from build123d import *

# Parameters (mm, degrees)
F0_W      = 127
F0_H      = 127
F1_DEPTH  = 127
F2_DEPTH  = 25.4
F3_DEPTH  = 76.2
F5_DEPTH  = 228.6
F6_W      = 55.9784695506
F6_H      = 69.2825764418
F7_DEPTH  = 5.08
F8_W      = 69.8941033334
F8_H      = 56.1961345005
F9_DEPTH  = 7.62
F11_W     = 69.8941033334
F11_H     = 56.1961345005
F10_W     = 69.8941033334
F10_H     = 56.1961345005
F12_DEPTH = 7.62
F13_T     = -5.08


# Not quite as in the source:
# - a shell that OpenCascade refuses in one call is made with other operations: the cavity is built on its own and cut out


with BuildPart() as f1:
    # F0 (on Top) → F1 (new body)
    with BuildSketch(Plane.XY):
        with Locations((63.5, -63.5)):
            Rectangle(F0_W, F0_H)
    extrude(amount=F1_DEPTH)

    # F2 (add): a face of the model
    f2_faces = [f1.faces().sort_by_distance(p)[0] for p in [
        (63.5, -127, 63.5),
    ]]
    extrude(f2_faces, amount=F2_DEPTH)

    # F3 (add): a face of the model
    f3_faces = [f1.faces().sort_by_distance(p)[0] for p in [
        (63.5, -152.4, 63.5),
    ]]
    extrude(f3_faces, amount=F3_DEPTH)

    # F4 (on face) → F5 (join)
    with BuildSketch(Plane.XZ.offset(228.6)):
        Polygon((63.5, 210.3958427906), (63.5, 127), (127, 127), align=None)
        Polygon((63.5, 210.3958427906), (0, 127), (63.5, 127), align=None)
    extrude(amount=-F5_DEPTH)

    # F6 (on face) → F7 (cut)
    with BuildSketch(Plane.XZ.offset(228.6)):
        with Locations((68.3894939721, 34.6412882209)):
            Rectangle(F6_W, F6_H)
    extrude(amount=-F7_DEPTH, mode=Mode.SUBTRACT)

    # F8 (on face) → F9 (cut)
    with BuildSketch(Plane(origin=(0, 0, 0), x_dir=(0, -1, 0), z_dir=(-1, 0, 0))):
        with Locations((55.1468739286, 62.0407964849)):
            Rectangle(F8_W, F8_H)
        with Locations((160.0488739286, 62.0407964849)):
            Rectangle(F8_W, F8_H)
    extrude(amount=-F9_DEPTH, mode=Mode.SUBTRACT)

    # F11 (on face) + F10 (on face) → F12 (cut)
    with BuildSketch(Plane.YZ.offset(127)):
        with Locations((-160.0488739286, 62.0407964849)):
            Rectangle(F11_W, F11_H)
    with BuildSketch(Plane.YZ.offset(127)):
        with Locations((-55.1468739286, 62.0407964849)):
            Rectangle(F10_W, F10_H)
    extrude(amount=-F12_DEPTH, mode=Mode.SUBTRACT)

    # F13: a shell. OpenCascade refuses it in one call, so the cavity is built on its own and cut out:
    # the body offset inwards by the wall thickness, plus a prism from it out through each open face.
    f13_core = offset(f1.part, amount=F13_T, kind=Kind.INTERSECTION, mode=Mode.PRIVATE)
    f13_exits = [f13_core.faces().sort_by_distance(p)[0] for p in [
        (63.434775, -112.87691, 5.08),
    ]]
    add(f13_core, mode=Mode.SUBTRACT)
    extrude(f13_exits, amount=-F13_T, mode=Mode.SUBTRACT)


solid = f1.part
The listing builds one solid part. Answer for the finished solid, in the listing's coordinates (mm). A direction names the side the tool comes from. Coordinates: 2 decimals unless noted, no trailing zeros. Loops run counter-clockwise (first coordinate to the right, second up) from the corner with the lowest first, then second, coordinate; pieces in that order, holes last.
1) Find section D-D on z = 18.5. Write down the section's boundary in (x, y).
2) Find section B-B on y = -205. Write down the section's boundary in (x, z).
3) Find the intervals of material crossed by L1, parallel to Y at x = 66, z = 24.5; L2, parallel to X at y = -43.5, z = 105.5; L3, parallel to Y at x = 53, z = 152.5, in increasing order.
4) Determine the mould class of faces 1 (the face through (118, -56, 28.863)), 2 (the face through (4, -125.102, 62)), 3 (the face through (114.3, -56, 63)) for opening direction Z: pulls with the +Z half, pulls with the -Z half, needs draft (parallel to the pull), parting line crosses it, or undercut.
5) A tool of negligible diameter and unlimited length cuts with its end or side. For faces 4 (the face through (4, -160, 90.139)), 5 (the face through (127, -113, 63)), 6 (the face through (118, -200.076, 62)), 7 (the face through (121.92, -116, 64)), 8 (the face through (123, -161, 33.943)), from which of +Z, -Z, +X, -X, +Y, -Y can it reach the whole face along a straight path? Write none if from no direction.
6) Flat-ended cylindrical pins translate along their axes: pin 1 Ø6 at (x, y) = (2.5, -67.5) entering from +Z; pin 2 Ø10 at (x, y) = (22.5, -95) entering from -Z; pin 3 Ø10 at (x, y) = (87.5, -97) entering from +Z. Find the tip coordinate at first contact, or state that the pin passes through.
7) Find section C-C on x = 93. Write down the section's boundary in (y, z).
8) Find section A-A on z = 110. Write down the section's boundary in (x, y), then the cut area to 3 significant figures.
Values:
1. outline: (0, -228.6) - (40.4, -228.6) - (40.4, -223.52) - (96.38, -223.52) - (96.38, -228.6) - (127, -228.6) - (127, 0) - (0, 0) - close; hole (5.08, -223.52) - (35.32, -223.52) - (35.32, -218.44) - (101.46, -218.44) - (101.46, -223.52) - (121.92, -223.52) - (121.92, -5.08) - (5.08, -5.08) - close
2. outline: (0, 0) - (5.08, 0) - (5.08, 125.29) - (63.5, 202.01) - (121.92, 125.29) - (121.92, 0) - (127, 0) - (127, 127) - (63.5, 210.4) - (0, 127) - close
3. L1: y = -223.52 to -218.44, -5.08 to 0
3. L2: x = 0 to 5.08, 121.92 to 127
3. L3: y = -228.6 to -223.52, -5.08 to 0
4. face 1: pulls with the -Z half
4. face 2: undercut
4. face 3: needs draft
5. face 4: -X
5. face 5: +Z, -Z, +X, +Y, -Y
5. face 6: -Z
5. face 7: none
5. face 8: +X
6. pin 1: stops at z = 134.22
6. pin 2: stops at z = 141.6
6. pin 3: stops at z = 185.44
7. outline: (-228.6, 69.28) - (-223.52, 69.28) - (-223.52, 0) - (-218.44, 0) - (-218.44, 74.36) - (-223.52, 74.36) - (-223.52, 163.27) - (-5.08, 163.27) - (-5.08, 0) - (0, 0) - (0, 171.65) - (-228.6, 171.65) - close
8. outline: (0, -228.6) - (127, -228.6) - (127, 0) - (0, 0) - close; hole (5.08, -223.52) - (121.92, -223.52) - (121.92, -5.08) - (5.08, -5.08) - close
8. area: 3,510 mm2
